The model under review builds one solid part; all positions refer to its coordinate system, in mm. A direction names the side the tool comes from. Round coordinates to 2 decimals unless told otherwise and drop trailing zeros. Loops run counter-clockwise (first coordinate to the right, second up) from the corner with the lowest first, then second, coordinate; pieces in that order, holes last. Notation, with made-up numbers: M 81.25,89 L 140.25,89 A13 ccw 140.25,101 Z; hole C -29,89.25 d9. An arc over 180 degrees is marked long. Return JSON: item names as keys, results as strings. Group by question number.
Q1. Consider section B-B (z = 8.5). State the section outline as (x, y) points.
Q2. Consider section D-D (x = 11.5). State the section outline as (y, z) points, and give its area (3 significant figures).
Q3. For faces 4 (the face through (3, 2, 10)), 5 (the face through (0, 5, 5)), list the 3-axis set-ups (+Z, -Z, +X, -X, +Y, -Y) from which the entire face can be reached by the end or side of a thin tool; tool diameter is ignored.
Q4. Clearance check with flat-ended pins moving along their axes: pin 1 Ø8 at (x, y) = (0, 0.5) entering from -Z; pin 2 Ø1.2 at (x, y) = (1, 0) entering from +Z. State where each tip first meets the part, or that it passes through.
Q5. Consider section C-C (y = -0.75). State the section outline as (x, z) points.
Q6. Consider section A-A (x = 5). State the section outline as (y, z) points, and give its area (3 significant figures).
Q7. To check wall thickness, follow line 1 along Y through (x, z) = (10, 7.3); line 2 along X through (y, z) = (0, 6.8); line 3 along X through (y, z) = (0.5, 8.25). State the ranges of each line that lie inside material, in increasing order.
Q8. Draft analysis for pull direction Y (two halves, no side actions). For faces 1 (the face through (5, 9, 5)), 2 (the face through (0, 0, 5)), 3 (the face through (-4, 2, 5)), state which applies: pulls with the +Y half, pulls with the -Y half, needs draft (parallel to the pull), parting line crosses it, or undercut.
from build123d import *

# Parameters (mm, degrees)
CYLINDER001_R     = 2
CYLINDER001_DEPTH = 10
CYLINDER002_R     = 2
CYLINDER002_DEPTH = 10
CYLINDER003_R     = 2
CYLINDER003_DEPTH = 10
CYLINDER004_R     = 2
CYLINDER004_DEPTH = 10
CYLINDER005_R     = 2
CYLINDER005_DEPTH = 10
CYLINDER_R        = 2
CYLINDER_DEPTH    = 10
BOX_W             = 18
BOX_H             = 14
BOX_DEPTH         = 10


with BuildPart() as cilindre2:
    # Cylinder001 → Cylinder001 (new body)
    with BuildSketch(Plane(origin=(0, 5, 5), x_dir=(1, 0, 0), z_dir=(0, 0, 1))):
        Circle(CYLINDER001_R)
    extrude(amount=CYLINDER001_DEPTH)


with BuildPart() as cilindre3:
    # Cylinder002 → Cylinder002 (new body)
    with BuildSketch(Plane(origin=(5, 5, 5), x_dir=(1, 0, 0), z_dir=(0, 0, 1))):
        Circle(CYLINDER002_R)
    extrude(amount=CYLINDER002_DEPTH)


with BuildPart() as cilindre4:
    # Cylinder003 → Cylinder003 (new body)
    with BuildSketch(Plane(origin=(5, 0, 5), x_dir=(1, 0, 0), z_dir=(0, 0, 1))):
        Circle(CYLINDER003_R)
    extrude(amount=CYLINDER003_DEPTH)


with BuildPart() as cilindre5:
    # Cylinder004 → Cylinder004 (new body)
    with BuildSketch(Plane(origin=(10, 0, 5), x_dir=(1, 0, 0), z_dir=(0, 0, 1))):
        Circle(CYLINDER004_R)
    extrude(amount=CYLINDER004_DEPTH)


with BuildPart() as cilindre6:
    # Cylinder005 → Cylinder005 (new body)
    with BuildSketch(Plane(origin=(10, 5, 5), x_dir=(1, 0, 0), z_dir=(0, 0, 1))):
        Circle(CYLINDER005_R)
    extrude(amount=CYLINDER005_DEPTH)


with BuildPart() as obj1:
    # Cylinder → Cylinder (new body)
    with BuildSketch(Plane.XY.offset(5)):
        Circle(CYLINDER_R)
    extrude(amount=CYLINDER_DEPTH)

    # Fusion: union cilindre2, cilindre3, cilindre4, cilindre5, cilindre6
    add(cilindre2.part)
    add(cilindre3.part)
    add(cilindre4.part)
    add(cilindre5.part)
    add(cilindre6.part)


with BuildPart() as cut:
    # Box → Box (new body)
    with BuildSketch(Plane(origin=(-4, -5, 0), x_dir=(1, 0, 0), z_dir=(0, 0, 1))):
        with Locations((9, 7)):
            Rectangle(BOX_W, BOX_H)
    extrude(amount=BOX_DEPTH)

    # Cut: cut obj1
    add(obj1.part, mode=Mode.SUBTRACT)


solid = cut.part
Values:
{
 "1": {"outline": "M -4,-5 L 14,-5 L 14,9 L -4,9 Z; hole C 0,0 d4; hole C 0,5 d4; hole C 5,0 d4; hole C 5,5 d4; hole C 10,0 d4; hole C 10,5 d4"},
 "2": {"outline": "M -5,0 L 9,0 L 9,10 L 6.32,10 L 6.32,5 L 3.68,5 L 3.68,10 L 1.32,10 L 1.32,5 L -1.32,5 L -1.32,10 L -5,10 Z", "area": "114 mm2"},
 "3": {"face 4": "+Z, +X, -X, +Y, -Y", "face 5": "+Z"},
 "4": {"pin 1": "stops at z = 0", "pin 2": "stops at z = 5"},
 "5": {"outline": "M -4,0 L 14,0 L 14,10 L 11.85,10 L 11.85,5 L 8.15,5 L 8.15,10 L 6.85,10 L 6.85,5 L 3.15,5 L 3.15,10 L 1.85,10 L 1.85,5 L -1.85,5 L -1.85,10 L -4,10 Z"},
 "6": {"outline": "M -5,0 L 9,0 L 9,10 L 7,10 L 7,5 L 3,5 L 3,10 L 2,10 L 2,5 L -2,5 L -2,10 L -5,10 Z", "area": "100 mm2"},
 "7": {"line 1": "y = -5 to -2, 2 to 3, 7 to 9", "line 2": "x = -4 to -2, 2 to 3, 7 to 8, 12 to 14", "line 3": "x = -4 to -1.94, 1.94 to 3.06, 6.94 to 8.06, 11.94 to 14"},
 "8": {"face 1": "pulls with the +Y half", "face 2": "undercut", "face 3": "needs draft"}
}
